Autodesk Inventor part; units mm, degrees
ref_plane "YZ Plane" through (0, 0, 0) normal (1, 0, 0) x (0, 1, 0)
ref_plane "XZ Plane" through (0, 0, 0) normal (0, 1, 0) x (-1, 0, 0)
ref_plane "XY Plane" through (0, 0, 0) normal (0, 0, 1) x (1, 0, 0)
sketch "Sketch1" plane through (0, 0, 0) normal (0, 0, 1) x (1, 0, 0)
  line L0 (65.5, 25) -> (-65.5, 25)
  line L1 (-65.5, 25) -> (-65.5, -25)
  line L2 (-65.5, -25) -> (65.5, -25)
  line L3 (65.5, -25) -> (65.5, 25)
  line L4 (65.5, 25) -> (-65.5, -25) construction
  line L5 (-65.5, 25) -> (65.5, -25) construction
  line L6 (0, 0) -> (-24.1, 0)
  line L7 (0, 0) -> (24.1, 0)
  circle A0 centre (-24.1, 0) radius 3.5
  circle A1 centre (24.1, 0) radius 3.5
  dimension "d0" = 131
  dimension "d1" = 50
  dimension "d2" = 24.1
  dimension "d3" = 24.1
  dimension "d4" = 7
  dimension "d5" = 7
extrude "Extrusion1" add sketch "Sketch1" along normal blind 10
properties part number "prepazka_bez_loziska"
Input: part model. Units: mm. Frame: model coordinates. Give positions to 0.01 mm unless a question says otherwise; leave off trailing zeros. Order: outer loops, then holes, each group sorted by start corner. A loop starts at its lowest first (then second) coordinate and runs counter-clockwise, first axis right, second up. Notation, with made-up numbers: M -18.5,23 L 13.5,23 A13 ccw 13.5,36 Z; hole C 82,68.25 d2. An arc over 180 degrees is marked long. Return JSON: item names as keys, results as strings.
Item 1: Cut plane A-A (x = -24.1). Return loops of the section in (y, z), then the cut area to 3 significant figures.
Solutions:
{"outline": "M -25,0 L -3.5,0 L -3.5,10 L -25,10 Z; M 3.5,0 L 25,0 L 25,10 L 3.5,10 Z", "area": "430 mm^2"}
Item 2: Pull-direction query (Y, two-part tool) for faces 1 (the flat face through (-1, 0, 0)), 2 (the cylindrical face through (21.52, -2.365, 4.93)), 3 (the flat face through (1, 25, 5)), 4 (the flat face through (-1, -25, 5)); classes: +Y half, -Y half, draft (parallel to the pull), parting line (faces both ways), or undercut.
Solutions:
{"face 1": "draft", "face 2": "undercut", "face 3": "+Y half", "face 4": "-Y half"}
Item 3: Ray query, probe 1 along Y at (x, z) = (-24.1, 7.25); probe 2 along X at (y, z) = (-2.5, 2.5). Return the intervals inside material, ascending.
Solutions:
{"probe 1": "-25 to -3.5, 3.5 to 25", "probe 2": "-65.5 to -26.55, -21.65 to 21.65, 26.55 to 65.5"}
Item 4: First-contact query: P1, Ø4, axis at x = 24.1, y = 0, coming from the -Z side. Flat tip, straight axial feed; report the tip coordinate or a pass-through.
Solutions:
{"P1": "through"}
Item 5: Cut plane B-B (y = 0). Return loops of the section in (x, z), then the cut area to 3 significant figures.
Solutions:
{"outline": "M -65.5,0 L -27.6,0 L -27.6,10 L -65.5,10 Z; M -20.6,0 L 20.6,0 L 20.6,10 L -20.6,10 Z; M 27.6,0 L 65.5,0 L 65.5,10 L 27.6,10 Z", "area": "1,170 mm^2"}
